The figure shows three views and two pictorial views of one solid part (mm, origin at its lowest corner). Answer the questions. Round coordinates to 2 decimals unless told otherwise and drop trailing zeros. Order: outer loops, then holes, each group sorted by start corner. A loop starts at its lowest first (then second) coordinate and runs counter-clockwise, first axis right, second up.
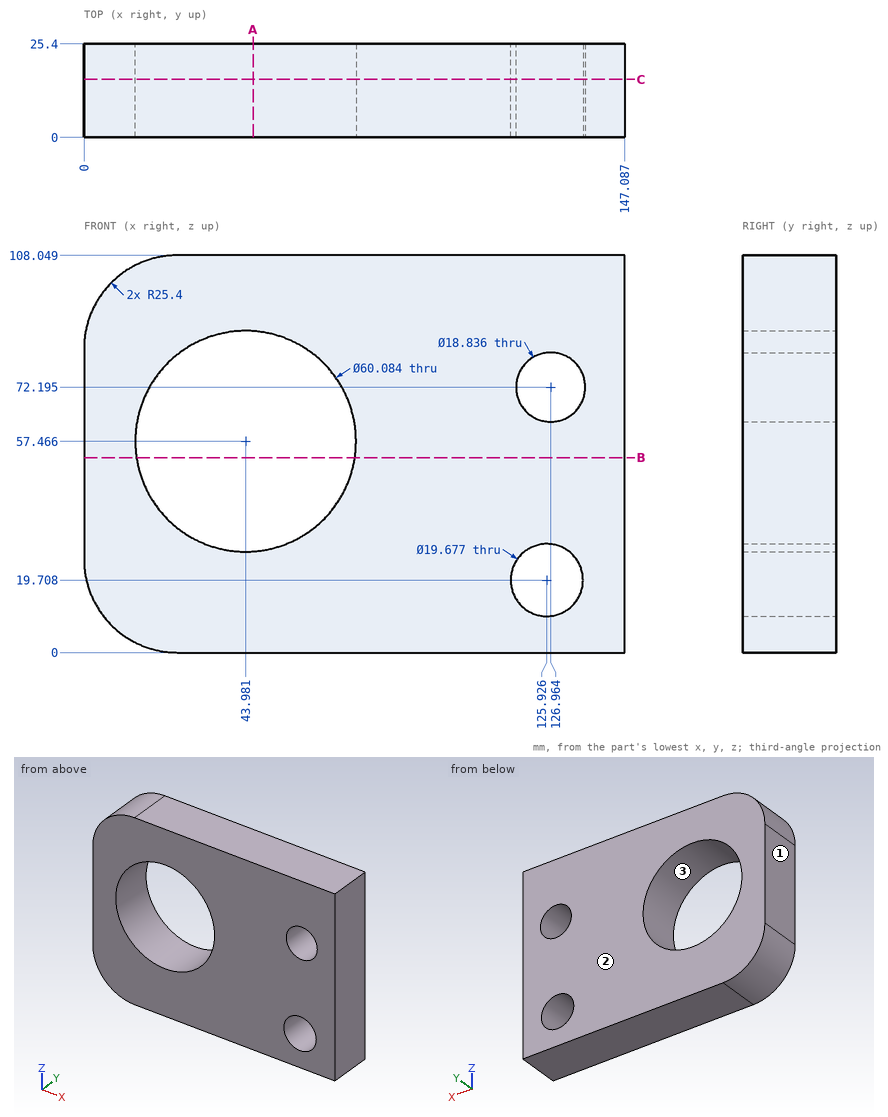
Item 1: For a pull along X with two mould halves and no side action, classify the marked faces 1, 2 and 3 as released by +X, released by -X, zero draft, split by the parting line, or undercut.
Item 2: Given pin 1 (17 mm diameter, centred on x = 126.96, z = 72.2, fed in from +Y), flat-ended and moving along its own axis, determine where the tip first touches the part or whether it passes through.
Item 3: Find section A-A (x = 46). Write down the section's boundary in (y, z), plus the area to 3 significant figures.
Item 4: Find section B-B (z = 53). Write down the section's boundary in (x, y), plus the area to 3 significant figures.
Item 5: Find section C-C (y = 15.75). State how many separate pieces and enclosed holes the cut face has, plus the area to 3 significant figures.
Item 6: Find the intervals of material crossed by line 1 along Z through (x, y) = (122, 23.5); line 2 along X through (y, z) = (7, 72); line 3 along X through (y, z) = (11.5, 57), in increasing order.
Model answer:
1. face 1: released by -X
1. face 2: zero draft
1. face 3: undercut
2. pin 1: passes through
3. outline: (0, 0) - (25.4, 0) - (25.4, 27.49) - (0, 27.49) - close; (0, 87.44) - (25.4, 87.44) - (25.4, 108.05) - (0, 108.05) - close
3. area: 1,220 mm2
4. outline: (0, 0) - (14.27, 0) - (14.27, 25.4) - (0, 25.4) - close; (73.69, 0) - (147.09, 0) - (147.09, 25.4) - (73.69, 25.4) - close
4. area: 2,230 mm2
5. separate pieces: 1
5. enclosed holes: 3
5. area: 12,200 mm2
6. line 1: z = 0 to 10.69, 28.73 to 64.19, 80.2 to 108.05
6. line 2: x = 0 to 17.69, 70.27 to 117.55, 136.38 to 147.09
6. line 3: x = 0 to 13.94, 74.02 to 147.09
